Source: CAD feature listing. Evaluate the final solid. Frame: model axes, mm. Face numbers are marked on the shaded views. A direction names the side the tool comes from. Round coordinates to 2 decimals unless told otherwise and drop trailing zeros. Loops run counter-clockwise (first coordinate to the right, second up) from the corner with the lowest first, then second, coordinate; pieces in that order, holes last. Notation, with made-up numbers: (38, 69) -> (64, 69) arc R21 ccw to (64, 82) -> close; hole circle Ø11 at (81, 89). An arc over 180 degrees is marked (long way). Write item = value, one per line.
Autodesk Inventor part; units mm, degrees
ref_plane "Plan de construction2" through (0, -8.75, 15.1554) normal (0, -0.5, 0.8660254) x (1, 0, 0)
ref_plane "Plan de construction4" through (0, -10, 10) normal (0, -0.7071068, 0.7071068) x (1, 0, 0)
ref_plane "YZ Plane" through (0, 0, 0) normal (1, 0, 0) x (0, 1, 0)
sketch "Esquisse1" plane through (0, 0, 0) normal (0, 0, 1) x (1, 0, 0)
  circle A0 centre (0, 0) radius 8
  circle A1 centre (0, 0) radius 9
  dimension "d0" = 16
  dimension "d1" = 18
extrude "Extrusion1" add sketch "Esquisse1" along normal blind 10
sketch "Esquisse2" plane through (0, 0, 0) normal (1, 0, 0) x (0, 1, 0)
  line L0 (9, 10) -> (-9, 10)
  line L1 (0, 10) -> (0, 25)
  line L2 (9, 10) -> (-9, 10)
  line L3 (0, 10) -> (10, 10)
  line L4 (10, 10) -> (10, 30)
  line L5 (10, 30) -> (-10, 30)
  line L6 (-10, 30) -> (-10, 10)
  line L7 (-10, 10) -> (0, 10)
  point P0 (0, 0)
  dimension "d26" = 10
  dimension "d27" = 20
  dimension "d28" = 20
  dimension "d29" = 90
extrude "Extrusion2" add sketch "Esquisse2" along normal mid plane 20
fillet "Congé1" radius 2 1 edges at (-9, 0, 10)
sketch "Esquisse4" plane through (0, 0, 0) normal (0, 1, 0) x (-1, 0, 0)
  line L0 (9, 0) -> (-9, 0)
  line L1 (9, 0) -> (0, 0)
  line L2 (0, 0) -> (0, 5)
  line L3 (0, 0) -> (5, 0) construction
  dimension "d14" = 9
  dimension "d15" = 5
  dimension "d16" = 90
hole "Perçage1" at (0, 0, 5) direction (0, -1, 0) diameter 4 end through all both
ref_plane "Plan de construction2" through (0, -8.75, 15.1554) normal (0, -0.5, 0.8660254) x (1, 0, 0)
ref_plane "Plan de construction1" through (0, 0, 0) normal (0, -0.5, 0.8660254) x (1, 0, 0)
ref_plane "Plan de construction4" through (0, -10, 10) normal (0, -0.7071068, 0.7071068) x (1, 0, 0)
ref_plane "Plan de construction3" through (0, 0, 0) normal (0, -0.7071068, 0.7071068) x (1, 0, 0)
sketch "Esquisse6" plane through (0, -10, 10) normal (0, -0.7071068, 0.7071068) x (1, 0, 0)
  line L0 (-10, 28.2843) -> (-10, 14.1421)
  line L1 (10, 14.1421) -> (10, 0)
  line L2 (-10, 28.2843) -> (10, 28.2843)
  line L3 (10, 28.2843) -> (10, 0)
  line L4 (10, 0) -> (-10, 0)
  line L5 (-10, 0) -> (-10, 28.2843)
  line L6 (-10, 28.2843) -> (10, 28.2843)
  line L7 (10, 14.1421) -> (10, 28.2843)
  line L8 (4.5826, 14.1421) -> (10, 14.1421)
  line L9 (-10, 14.1421) -> (-4.5826, 14.1421)
  line L10 (-10, 28.2843) -> (-10, 14.1421)
  point P0 (0, 0)
extrude "Extrusion4" add sketch "Esquisse6" along normal blind 25
sketch "Esquisse8" plane through (-10, 10, 30) normal (0, 0.7071068, 0.7071068) x (1, 0, 0)
  line L0 (20, 0) -> (0, 0)
  line L1 (0, 0) -> (0, -25)
  line L2 (20, -25) -> (0, -25)
  line L3 (20, 0) -> (20, -25)
  point P0 (10, 14.1422)
extrude "Extrusion5" add sketch "Esquisse8" along normal blind 40
fillet "Congé4" radius 20 1 edges at (0, -27.6777, 27.6777)
fillet "Congé5" radius 10 2 edges at (0, 38.2842, 58.2843) (0, 20.6066, 75.962)
sketch "Esquisse9" plane through (10, 0, 0) normal (1, 0, 0) x (0, 0, -1)
  line L0 (-41.8199, -13.5356) -> (-68.8909, 13.5355)
  line L1 (-30, 9.9999) -> (-51.2132, 31.2132)
  line L2 (-68.8909, 27.6776) -> (-65.3554, 31.2132)
  arc A0 (-68.8909, 27.6776) -> (-68.8909, 13.5355) centre (-61.8199, 20.6066) ccw
  circle A1 centre (-53.9284, 16.2506) radius 4.25
  point P0 (0, 0)
  point P1 (-67.1232, 29.4454)
  point P2 (-71.8199, 20.6066)
  dimension "d48" = 8.5
extrude "Extrusion6" cut sketch "Esquisse9" against normal through all
sketch "Esquisse10" plane through (10, 0, 0) normal (1, 0, 0) x (0, 0, -1)
  circle A0 centre (-53.9284, 16.2506) radius 4.25
  circle A1 centre (-53.9284, 16.2506) radius 7.5
  circle A2 centre (-53.9284, 16.2506) radius 10.95
  point P0 (0, 0)
  dimension "d49" = 15
  dimension "d50" = 21.9
extrude "Extrusion7" add sketch "Esquisse10" along normal blind 3 contours A2
sketch "Esquisse11" plane through (10, 0, 0) normal (1, 0, 0) x (0, 0, -1)
  circle A0 centre (-53.9284, 16.2506) radius 10.95
  circle A1 centre (-53.9284, 16.2506) radius 7.5
  circle A2 centre (-53.9284, 16.2506) radius 4.25
  circle A3 centre (-53.9284, 16.2506) radius 12.5
  line L0 (-30, 9.9999) -> (-51.2132, 31.2132)
  point P0 (0, 0)
extrude "Extrusion8" add sketch "Esquisse11" along normal blind 2 contours A0 | A3
properties part number "bielle roue milieu"
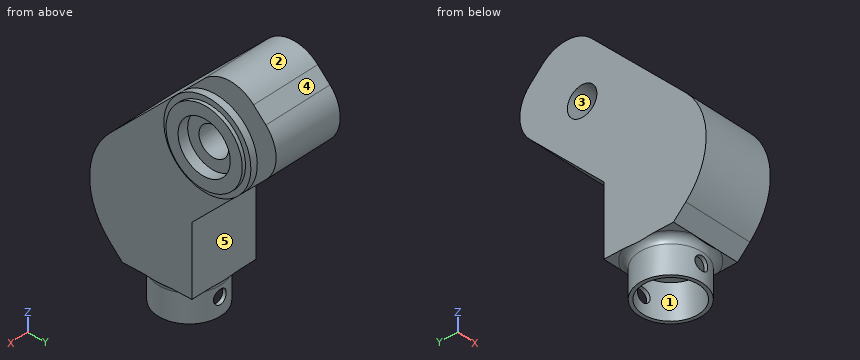
1. Contact query for flat-ended pins moving along their axis: pin 1 Ø13.5 at (y, z) = (16.25, 53.93) entering from -X; pin 2 Ø2 at (x, y) = (5, 11) entering from +Z; pin 3 Ø1.5 at (x, z) = (10.5, 11) entering from -Y; pin 4 Ø6 at (x, z) = (3, 8.5) entering from -Y. Output: stop coordinate, or through.
Evaluation:
pin_1 = -10
pin_2 = 67.36
pin_3 = -11.56
pin_4 = -11.5
2. Section query D-D (z = 55). Return the cut outline in (x, y), then the cut area to 3 significant figures.
Evaluation:
outline = (-10, -0.36) -> (10, -0.36) -> (10, 3.8) -> (12, 3.8) -> (12, 5.35) -> (13, 5.35) -> (13, 8.83) -> (10, 8.83) -> (10, 12.14) -> (-10, 12.14) -> close; (-10, 20.36) -> (10, 20.36) -> (10, 23.67) -> (13, 23.67) -> (13, 27.15) -> (12, 27.15) -> (12, 28.7) -> (10, 28.7) -> (10, 33.59) -> (-10, 33.59) -> close
area = 541 mm²
3. Line query: probe 1 along Z at (x, y) = (0, -8.4); probe 2 along X at (y, z) = (-8, 5); probe 3 along X at (y, z) = (-2, 28). Output: solid intervals per line, ascending. Write a range as from..to.
Evaluation:
probe_1 = 0..3, 7..46.96
probe_2 = -4.12..-2, 2..4.12
probe_3 = -10..10
4. Section query A-A (x = 0). Return the cut outline in (y, z).
Evaluation:
outline = (-13.54, 13.54) -> (-10, 10) -> (-10, 9.73) arc R2 cw to (-9, 8) -> (-9, 7) -> (-8, 7) -> (-8, 10) -> (8, 10) -> (8, 7) -> (9, 7) -> (9, 8) arc R2 cw to (10, 9.73) -> (10, 30) -> (31.21, 51.21) arc R10 ccw to (31.21, 65.36) -> (27.68, 68.89) arc R10 ccw to (13.54, 68.89) -> (-13.54, 41.82) arc R20 ccw to start; (-9, 0) -> (-8, 0) -> (-8, 3) -> (-9, 3) -> close; (8, 0) -> (9, 0) -> (9, 3) -> (8, 3) -> close; hole circle Ø8.5 at (16.25, 53.93)
5. Set-up query: the marked faces 1 and 2. Return all of +Z, -Z, +X, -X, +Y, -Y with unobstructed straight access to the full face (end or side cutting, diameter ignored); none if empty.
Evaluation:
face_1 = -Z
face_2 = +Z, +X, -X
6. Mould query, pull axis Z, two halves, no side actions, for the marked faces 3, 4 and 5. Classes: released by +Z, released by -Z, zero draft, split by the parting line, or undercut.
Evaluation:
face_3 = undercut
face_4 = released by +Z
face_5 = zero draft
7. Section query C-C (y = 0). Return the cut outline in (x, z), then the cut area to 3 significant figures.
Evaluation:
outline = (-10, 9.73) arc R2 cw to (-9, 8) -> (-9, 0) -> (-8, 0) -> (-8, 10) -> (8, 10) -> (8, 0) -> (9, 0) -> (9, 8) arc R2 cw to (10, 9.73) -> (10, 55.36) -> (-10, 55.36) -> close
area = 929 mm²
